from build123d import *

# Parameters (mm, degrees)
PAD_DEPTH    = 12
SKETCH001_R  = 2.1
POCKET_DEPTH = 5


with BuildPart() as part:
    # Sketch → Pad (new body)
    with BuildSketch(Plane.XY):
        with BuildLine():
            Line((0, 48.5), (3.5, 48.5))
            Line((3.5, 48.5), (3.5, -48.5))
            Line((3.5, -48.5), (0, -48.5))
            Line((0, -48.5), (-7, -48.5))
            ThreePointArc((-7, -38.5), (-12, -43.5), (-7, -48.5))
            Line((-7, -38.5), (0, -38.5))
            Line((0, 38.5), (0, -38.5))
            Line((-7, 38.5), (0, 38.5))
            ThreePointArc((-7, 48.5), (-12, 43.5), (-7, 38.5))
            Line((0, 48.5), (-7, 48.5))
        make_face()
        Polygon((-4.120352, 41.790917), (-4.080067, 45.139307), (-6.959715, 46.848389), (-9.879648, 45.209083), (-9.919933, 41.860693), (-7.040285, 40.151611), align=None, mode=Mode.SUBTRACT)
        Polygon((-4.1, -45.174316), (-4.1, -41.825684), (-7, -40.151368), (-9.9, -41.825684), (-9.9, -45.174316), (-7, -46.848632), align=None, mode=Mode.SUBTRACT)
    extrude(amount=PAD_DEPTH)

    # Sketch001 (on Face3 of Pad) → Pocket (cut)
    with BuildSketch(Plane.YZ.offset(3.5)):
        with Locations((-30, 6)):
            Circle(SKETCH001_R)
        with Locations((30, 6)):
            Circle(SKETCH001_R)
    extrude(amount=-POCKET_DEPTH, mode=Mode.SUBTRACT)


solid = part.part
Design review of the part built by this model. Coordinates are the model's own, in mm. A direction names the side the tool comes from. Round coordinates to 2 decimals unless told otherwise and drop trailing zeros. Write each loop counter-clockwise with the first axis right and the second up, starting at its lowest first coordinate (ties: lowest second). Pieces come first, ordered by that corner, then holes. Notation, with made-up numbers: M 10,-8.5 L 18,-8.5 A15 cw 18,18.5 Z; hole C 7,-32 d10. An arc over 180 degrees is marked long. One line per item, written item: value. Start each with the question number.
1. To check wall thickness, follow probe 1 along Z at (x, y) = (0.75, 30); probe 2 along Y at (x, z) = (-6.75, 10); probe 3 along Y at (x, z) = (-1, 2.5). State the ranges of each line that lie inside material, in increasing order. Write a range as from..to.
2. Take a section at C-C on z = 1.5. State the section outline as (x, y) points, then the cut area to 3 significant figures.
3. Clearance check with flat-ended pins moving along their axes: P1, Ø6, axis at y = 4.5, z = 7, coming from the -X side; P2, Ø3.5, axis at y = 30, z = 6, coming from the +X side. State where each tip first meets the part, or that it passes through.
4. Take a section at A-A on y = -30. State the section outline as (x, z) points, then the cut area to 3 significant figures.
5. Take a section at D-D on x = -5.5. State the section outline as (y, z) points, then the cut area to 3 significant figures.
6. Draft analysis for pull direction Z (two halves, no side actions). For faces 4 (the face through (-12, 43.6, 5.9)), 5 (the face through (1.77, 27.9, 6.09)), 6 (the face through (0.4, 0.2, 0)), state which applies: pulls with the +Z half, pulls with the -Z half, needs draft (parallel to the pull), parting line crosses it, or undercut.
7. For faces 1 (the face through (-2, -48.5, 6)), 2 (the face through (0, 1, 6)), 3 (the face through (-5.6, 40.96, 5.92)), list the 3-axis set-ups (+Z, -Z, +X, -X, +Y, -Y) from which the entire face can be reached by the end or side of a thin tool; tool diameter is ignored.
8. Take a section at B-B on z = 6. State the section outline as (x, y) points, then the cut area to 3 significant figures.
Computed:
1. probe 1: z = 0..3.9, 8.1..12
1. probe 2: y = -48.5..-46.7, -40.3..-38.5, 38.5..40.31, 46.72..48.5
1. probe 3: y = -48.5..-38.5, 38.5..48.5
2. outline: M -7,-48.5 L 3.5,-48.5 L 3.5,48.5 L -7,48.5 A5 ccw -7,38.5 L 0,38.5 L 0,-38.5 L -7,-38.5 A5 ccw Z; hole M -9.92,41.86 L -7.04,40.15 L -4.12,41.79 L -4.08,45.14 L -6.96,46.85 L -9.88,45.21 Z; hole M -9.9,-45.17 L -7,-46.85 L -4.1,-45.17 L -4.1,-41.83 L -7,-40.15 L -9.9,-41.83 Z
2. area: 500 mm²
3. P1: stops at x = 0
3. P2: passes through
4. outline: M 0,0 L 3.5,0 L 3.5,3.9 L 0,3.9 Z; M 0,8.1 L 3.5,8.1 L 3.5,12 L 0,12 Z
4. area: 27.3 mm²
5. outline: M -48.5,0 L -45.98,0 L -45.98,12 L -48.5,12 Z; M -41.02,0 L -38.5,0 L -38.5,12 L -41.02,12 Z; M 38.5,0 L 41.02,0 L 41.02,12 L 38.5,12 Z; M 45.98,0 L 48.5,0 L 48.5,12 L 45.98,12 Z
5. area: 121 mm²
6. face 4: needs draft
6. face 5: undercut
6. face 6: pulls with the -Z half
7. face 1: +Z, -Z, +X, -X, -Y
7. face 2: +Z, -Z, -X
7. face 3: +Z, -Z
8. outline: M -7,-48.5 L 3.5,-48.5 L 3.5,-32.1 L 0,-32.1 L 0,-38.5 L -7,-38.5 A5 ccw Z; M -7,38.5 L 0,38.5 L 0,32.1 L 3.5,32.1 L 3.5,48.5 L -7,48.5 A5 ccw Z; M 0,-27.9 L 3.5,-27.9 L 3.5,27.9 L 0,27.9 Z; hole M -9.92,41.86 L -7.04,40.15 L -4.12,41.79 L -4.08,45.14 L -6.96,46.85 L -9.88,45.21 Z; hole M -9.9,-45.17 L -7,-46.85 L -4.1,-45.17 L -4.1,-41.83 L -7,-40.15 L -9.9,-41.83 Z
8. area: 470 mm²
